CAD build for the part. Positions are in the model's coordinates, mm. Coordinates: 2 decimals unless noted, no trailing zeros. Order: outer loops, then holes, each group sorted by start corner. A loop starts at its lowest first (then second) coordinate and runs counter-clockwise, first axis right, second up. Notation, with made-up numbers: M 23.5,30.5 L 79.5,30.5 A18 cw 79.5,63.5 Z; hole C 77.5,-26 d11. An arc over 180 degrees is marked long. One line per item, written item: value.
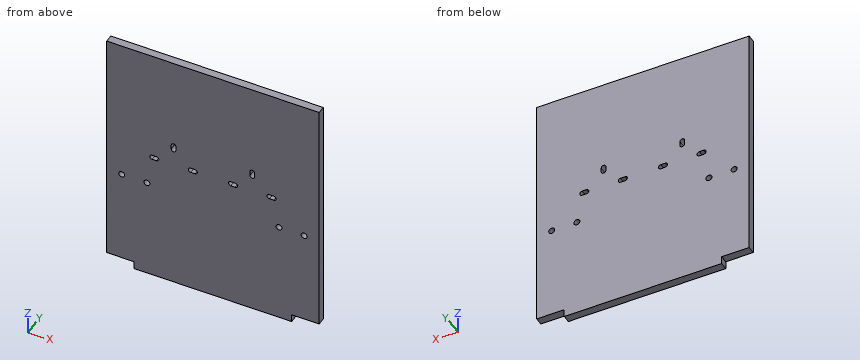
Autodesk Inventor part; units mm, degrees
ref_plane "YZ Plane" through (0, 0, 0) normal (1, 0, 0) x (0, 1, 0)
ref_plane "XZ Plane" through (0, 0, 0) normal (0, 1, 0) x (-1, 0, 0)
ref_plane "XY Plane" through (0, 0, 0) normal (0, 0, 1) x (1, 0, 0)
sketch "Sketch1" plane through (0, 0, 0) normal (0, 1, 0) x (-1, 0, 0)
  line L0 (-135, 160) -> (135, 160)
  line L1 (135, 160) -> (135, -160)
  line L2 (135, -160) -> (-135, -160)
  line L3 (-135, -160) -> (-135, 160)
  line L4 (-135, 160) -> (135, -160) construction
  line L5 (135, 160) -> (-135, -160) construction
  point P0 (0, 0)
  dimension "d0" = 270
  dimension "d1" = 320
extrude "Extrusion1" add sketch "Sketch1" along normal blind 10
sketch "Sketch2" plane through (0, 10, 0) normal (0, 1, 0) x (1, 0, 0)
  line L0 (57, -25.5) -> (57, -50)
  line L1 (57, -25.5) -> (43, -25.5)
  line L2 (43, -50) -> (43, -25.5)
  line L3 (57, -50) -> (43, -50)
  arc A0 (53, -33.75) -> (47, -33.75) centre (50, -33.75) ccw
  line L4 (53, -39.25) -> (53, -33.75)
  arc A1 (47, -39.25) -> (53, -39.25) centre (50, -39.25) ccw
  line L5 (47, -33.75) -> (47, -39.25)
  line L6 (63.5, -5) -> (88, -5)
  line L7 (63.5, -5) -> (63.5, -19)
  line L8 (88, -19) -> (63.5, -19)
  line L9 (88, -5) -> (88, -19)
  arc A2 (71.75, -9) -> (71.75, -15) centre (71.75, -12) ccw
  line L10 (77.25, -9) -> (71.75, -9)
  arc A3 (77.25, -15) -> (77.25, -9) centre (77.25, -12) ccw
  line L11 (71.75, -15) -> (77.25, -15)
  line L12 (36.5, -19) -> (12, -19)
  line L13 (36.5, -19) -> (36.5, -5)
  line L14 (12, -5) -> (36.5, -5)
  line L15 (12, -19) -> (12, -5)
  arc A4 (28.25, -15) -> (28.25, -9) centre (28.25, -12) ccw
  line L16 (22.75, -15) -> (28.25, -15)
  arc A5 (22.75, -9) -> (22.75, -15) centre (22.75, -12) ccw
  line L17 (28.25, -9) -> (22.75, -9)
  line L18 (-36.5, -5) -> (-12, -5)
  line L19 (-36.5, -5) -> (-36.5, -19)
  line L20 (-12, -19) -> (-36.5, -19)
  line L21 (-12, -5) -> (-12, -19)
  arc A6 (-28.25, -9) -> (-28.25, -15) centre (-28.25, -12) ccw
  line L22 (-22.75, -9) -> (-28.25, -9)
  arc A7 (-22.75, -15) -> (-22.75, -9) centre (-22.75, -12) ccw
  line L23 (-28.25, -15) -> (-22.75, -15)
  line L24 (-43, -25.5) -> (-43, -50)
  line L25 (-43, -25.5) -> (-57, -25.5)
  line L26 (-57, -50) -> (-57, -25.5)
  line L27 (-43, -50) -> (-57, -50)
  arc A8 (-47, -33.75) -> (-53, -33.75) centre (-50, -33.75) ccw
  line L28 (-47, -39.25) -> (-47, -33.75)
  arc A9 (-53, -39.25) -> (-47, -39.25) centre (-50, -39.25) ccw
  line L29 (-53, -33.75) -> (-53, -39.25)
  line L30 (-63.5, -19) -> (-88, -19)
  line L31 (-63.5, -19) -> (-63.5, -5)
  line L32 (-88, -5) -> (-63.5, -5)
  line L33 (-88, -19) -> (-88, -5)
  arc A10 (-71.75, -15) -> (-71.75, -9) centre (-71.75, -12) ccw
  line L34 (-77.25, -15) -> (-71.75, -15)
  arc A11 (-77.25, -9) -> (-77.25, -15) centre (-77.25, -12) ccw
  line L35 (-71.75, -9) -> (-77.25, -9)
  line L36 (-108.92, 42.1) -> (-108.92, 39.2309)
  line L37 (-108.52, 39) -> (-108.92, 39.2309)
  line L38 (-108.92, 38.7691) -> (-108.52, 39)
  line L39 (-108.92, 38.7691) -> (-108.92, 35.0867)
  line L40 (-108.92, 35.0867) -> (-117.2017, 32.9363)
  arc A12 (-117.2017, 32.9363) -> (-117.2017, 23.0637) centre (-115.92, 28) ccw
  line L41 (-117.2017, 23.0637) -> (-101.7351, 19.0476)
  arc A13 (-101.7351, 19.0476) -> (-100.579, 18.9) centre (-100.579, 23.5) ccw
  line L42 (-100.579, 18.9) -> (-99.2609, 18.9)
  arc A14 (-99.2609, 18.9) -> (-98.1048, 19.0476) centre (-99.2609, 23.5) ccw
  line L43 (-98.1048, 19.0476) -> (-82.6382, 23.0637)
  arc A15 (-82.6382, 23.0637) -> (-82.6382, 32.9363) centre (-83.92, 28) ccw
  line L44 (-82.6382, 32.9363) -> (-90.92, 35.0867)
  line L45 (-90.92, 42.1) -> (-90.92, 35.0867)
  line L46 (-90.92, 42.1) -> (-99.195, 42.1)
  line L47 (-99.195, 32.3399) -> (-99.195, 42.1)
  arc A16 (-100.645, 32.3399) -> (-99.195, 32.3399) centre (-99.92, 28) ccw
  line L48 (-100.645, 32.3399) -> (-100.645, 42.1)
  line L49 (-100.645, 42.1) -> (-108.92, 42.1)
  circle A17 centre (-115.92, 28) radius 3.8
  circle A18 centre (-83.92, 28) radius 3.8
  line L50 (90.92, 42.1) -> (90.92, 39.2309)
  line L51 (91.32, 39) -> (90.92, 39.2309)
  line L52 (90.92, 38.7691) -> (91.32, 39)
  line L53 (90.92, 38.7691) -> (90.92, 35.0867)
  line L54 (90.92, 35.0867) -> (82.6382, 32.9363)
  arc A19 (82.6382, 32.9363) -> (82.6382, 23.0637) centre (83.92, 28) ccw
  line L55 (82.6382, 23.0637) -> (98.1048, 19.0476)
  arc A20 (98.1048, 19.0476) -> (99.2609, 18.9) centre (99.2609, 23.5) ccw
  line L56 (99.2609, 18.9) -> (100.579, 18.9)
  arc A21 (100.579, 18.9) -> (101.7351, 19.0476) centre (100.579, 23.5) ccw
  line L57 (101.7351, 19.0476) -> (117.2017, 23.0637)
  arc A22 (117.2017, 23.0637) -> (117.2017, 32.9363) centre (115.92, 28) ccw
  line L58 (117.2017, 32.9363) -> (108.92, 35.0867)
  line L59 (108.92, 42.1) -> (108.92, 35.0867)
  line L60 (108.92, 42.1) -> (100.645, 42.1)
  line L61 (100.645, 32.3399) -> (100.645, 42.1)
  arc A23 (99.195, 32.3399) -> (100.645, 32.3399) centre (99.92, 28) ccw
  line L62 (99.195, 32.3399) -> (99.195, 42.1)
  line L63 (99.195, 42.1) -> (90.92, 42.1)
  circle A24 centre (83.92, 28) radius 3.8
  circle A25 centre (115.92, 28) radius 3.8
  point P0 (0, 0)
extrude "Extrusion2" cut sketch "Sketch2" against normal blind 10 contours L4 A1 L5 A0 | L10 A3 L11 A2 | L16 A5 L17 A4 | L22 A7 L23 A6 | L28 A9 L29 A8 | L34 A11 L35 A10 | A17 | A18 | A24 | A25
sketch "Sketch3" plane through (0, 10, 0) normal (0, 1, 0) x (1, 0, 0)
  arc A0 (-77.25, -9) -> (-77.25, -15) centre (-77.25, -12) ccw
  line L0 (-77.25, -9) -> (-71.75, -9)
  arc A1 (-71.75, -15) -> (-71.75, -9) centre (-71.75, -12) ccw
  line L1 (-71.75, -15) -> (-77.25, -15)
  circle A2 centre (83.92, 28) radius 3.8
  circle A3 centre (-115.92, 28) radius 3.8
  arc A4 (77.25, -15) -> (77.25, -9) centre (77.25, -12) ccw
  line L2 (77.25, -15) -> (71.75, -15)
  arc A5 (71.75, -9) -> (71.75, -15) centre (71.75, -12) ccw
  line L3 (71.75, -9) -> (77.25, -9)
  arc A6 (-22.75, -15) -> (-22.75, -9) centre (-22.75, -12) ccw
  line L4 (-22.75, -15) -> (-28.25, -15)
  arc A7 (-28.25, -9) -> (-28.25, -15) centre (-28.25, -12) ccw
  line L5 (-28.25, -9) -> (-22.75, -9)
  arc A8 (47, -39.25) -> (53, -39.25) centre (50, -39.25) ccw
  line L6 (47, -39.25) -> (47, -33.75)
  arc A9 (53, -33.75) -> (47, -33.75) centre (50, -33.75) ccw
  line L7 (53, -33.75) -> (53, -39.25)
  circle A10 centre (115.92, 28) radius 3.8
  circle A11 centre (-83.92, 28) radius 3.8
  arc A12 (22.75, -9) -> (22.75, -15) centre (22.75, -12) ccw
  line L8 (22.75, -9) -> (28.25, -9)
  arc A13 (28.25, -15) -> (28.25, -9) centre (28.25, -12) ccw
  line L9 (28.25, -15) -> (22.75, -15)
  arc A14 (-53, -39.25) -> (-47, -39.25) centre (-50, -39.25) ccw
  line L10 (-53, -39.25) -> (-53, -33.75)
  arc A15 (-47, -33.75) -> (-53, -33.75) centre (-50, -33.75) ccw
  line L11 (-47, -33.75) -> (-47, -39.25)
  line L12 (135, 160) -> (-135, 160)
  line L13 (-135, 160) -> (-135, -160)
  line L14 (-135, -160) -> (135, -160)
  line L15 (135, -160) -> (135, 160)
  line L16 (100, 170) -> (-100, 170)
  line L17 (-100, 170) -> (-100, 150)
  line L18 (-100, 150) -> (100, 150)
  line L19 (100, 150) -> (100, 170)
  line L20 (135, 160) -> (-135, 160)
  line L21 (100, 170) -> (-100, 150) construction
  line L22 (-100, 170) -> (100, 150) construction
  line L23 (-100, 150) -> (-135, 150)
  line L24 (-135, 160) -> (-135, -160)
  line L25 (100, 150) -> (135, 150)
  point P0 (0, 0)
  point P1 (0, 160)
  point P2 (-100, 160)
  point P3 (100, 160)
  dimension "d6" = 10
  dimension "d7" = 200
extrude "Extrusion3" cut sketch "Sketch3" against normal blind 49.25 contours L15 L25 L19 L12 | L17 L23 L13 L12
properties part number "12_Tam_go_top" material "Glass"
Q1. Pin check, flat tips, straight feed: pin 1 Ø4 at (x, y) = (-105, 7) entering from -Z; pin 2 Ø5 at (y, z) = (2.5, -157) entering from -X. Stop position of each tip, or through.
Recorded:
pin 1: stops at z = -150
pin 2: stops at x = -100
Q2. Slice it at B-B (x = -83.92). List the corners of the cut face in (y, z).
Recorded:
outline: M 0,-160 L 10,-160 L 10,-31.8 L 0,-31.8 Z; M 0,-24.2 L 10,-24.2 L 10,160 L 0,160 Z
Q3. Drill centre lines: line 1 along X through (y, z) = (4, -28); line 2 along Z through (x, y) = (-83.92, 2.25); line 3 along Z through (x, y) = (-72, 3.75). Where is each one in solid material? Low to high.
Recorded:
line 1: x = -135 to -119.72, -112.12 to -87.72, -80.12 to 80.12, 87.72 to 112.12, 119.72 to 135
line 2: z = -160 to -31.8, -24.2 to 160
line 3: z = -160 to 9, 15 to 160
Q4. Slice it at C-C (x = 108.5). List the corners of the cut face in (y, z), plus the area to 3 significant figures.
Recorded:
outline: M 0,-150 L 10,-150 L 10,160 L 0,160 Z
area: 3,100 mm^2
Q5. Slice it at A-A (x = -115.92). List the corners of the cut face in (y, z).
Recorded:
outline: M 0,-150 L 10,-150 L 10,-31.8 L 0,-31.8 Z; M 0,-24.2 L 10,-24.2 L 10,160 L 0,160 Z
